For this review, take the finished solid that the model builds, in its own axes (mm). A direction names the side the tool comes from. Coordinates: 2 decimals unless noted, no trailing zeros. Order: outer loops, then holes, each group sorted by start corner. A loop starts at its lowest first (then second) coordinate and runs counter-clockwise, first axis right, second up. Notation, with made-up numbers: M 54.25,52 L 97.25,52 A16 ccw 97.25,62 Z; hole C 89,83 d8. An arc over 180 degrees is marked long. Use CSV: the item, a comma, the result in double quotes.
```python
from build123d import *

# Parameters (mm, degrees)
SKETCH1_W           = 25.4
SKETCH1_H           = 12.7
BOSS_EXTRUDE1_DEPTH = 3.048
SKETCH2_W           = 3.048
SKETCH2_H           = 12.7
BOSS_EXTRUDE2_DEPTH = 15.875
SKETCH3_R           = 2.38125
CUT_EXTRUDE1_DEPTH  = 4.048
SKETCH4_R           = 2.38125
CUT_EXTRUDE2_DEPTH  = 4.048


with BuildPart() as part:
    # Sketch1 → Boss-Extrude1 (new body)
    with BuildSketch(Plane.XY):
        with Locations((12.7, 6.35)):
            Rectangle(SKETCH1_W, SKETCH1_H)
    extrude(amount=BOSS_EXTRUDE1_DEPTH)

    # Sketch2 → Boss-Extrude2 (add)
    with BuildSketch(Plane.XY.offset(3.048)):
        with Locations((1.524, 6.35)):
            Rectangle(SKETCH2_W, SKETCH2_H)
    extrude(amount=-BOSS_EXTRUDE2_DEPTH)

    # Sketch3 → Cut-Extrude1 (cut, through all)
    with BuildSketch(Plane(origin=(0, 0, 0), x_dir=(-1, 0, 0), z_dir=(0, 0, -1))):
        with Locations((-16.271875, 6.35)):
            Circle(SKETCH3_R)
    extrude(amount=-CUT_EXTRUDE1_DEPTH, mode=Mode.SUBTRACT)

    # Sketch4 → Cut-Extrude2 (cut, through all)
    with BuildSketch(Plane(origin=(3.048, 0, 0), x_dir=(0, 0, -1), z_dir=(1, 0, 0))):
        with Locations((4.8895, 6.35)):
            Circle(SKETCH4_R)
    extrude(amount=-CUT_EXTRUDE2_DEPTH, mode=Mode.SUBTRACT)


solid = part.part
```
Item 1: For faces 1 (the face through (0, 3, -5)), 2 (the face through (14, 5, 0)), list the 3-axis set-ups (+Z, -Z, +X, -X, +Y, -Y) from which the entire face can be reached by the end or side of a thin tool; tool diameter is ignored.
Solutions:
face 1,"+Z, -Z, -X, +Y, -Y"
face 2,"-Z, +X, +Y, -Y"
Item 2: Draft analysis for pull direction X (two halves, no side actions). For faces 3 (the face through (25.4, 6, 2)), 4 (the face through (16.788, 4.025, 1.503)), 5 (the face through (1.55, 5.44, -7.09)), state which applies: released by +X, released by -X, zero draft, split by the parting line, or undercut.
Solutions:
face 3,"released by +X"
face 4,"undercut"
face 5,"zero draft"
Item 3: Add section B-B on z = -6.75. State the section outline as (x, y) points, and give its area (3 significant figures).
Solutions:
outline,"M 0,0 L 3.05,0 L 3.05,4.86 L 0,4.86 Z; M 0,7.84 L 3.05,7.84 L 3.05,12.7 L 0,12.7 Z"
area,"29.6 mm^2"
Item 4: Add section A-A on y = 6.35. State the section outline as (x, z) points.
Solutions:
outline,"M 0,-12.83 L 3.05,-12.83 L 3.05,-7.27 L 0,-7.27 Z; M 0,-2.51 L 3.05,-2.51 L 3.05,0 L 13.89,0 L 13.89,3.05 L 0,3.05 Z; M 18.65,0 L 25.4,0 L 25.4,3.05 L 18.65,3.05 Z"
Item 5: To check wall thickness, follow line 1 along X through (y, z) = (2, -1.25); line 2 along X through (y, z) = (4.75, 0.5). State the ranges of each line that lie inside material, in increasing order. Write a range as [from, to].
Solutions:
line 1,"[0, 3.05]"
line 2,"[0, 14.51], [18.04, 25.4]"
Item 6: Add section D-D on y = 8. State the section outline as (x, z) points, and give its area (3 significant figures).
Solutions:
outline,"M 0,-12.83 L 3.05,-12.83 L 3.05,-6.61 L 0,-6.61 Z; M 0,-3.17 L 3.05,-3.17 L 3.05,0 L 14.55,0 L 14.55,3.05 L 0,3.05 Z; M 17.99,0 L 25.4,0 L 25.4,3.05 L 17.99,3.05 Z"
area,"95.6 mm^2"
Item 7: Add section C-C on x = 23.75. State the section outline as (y, z) points, and give its area (3 significant figures).
Solutions:
outline,"M 0,0 L 12.7,0 L 12.7,3.05 L 0,3.05 Z"
area,"38.7 mm^2"
